```python
from build123d import *

# Parameters (mm, degrees)
BOSS_EXTRU_1_DEPTH      = 25
ESQUISSE6_W             = 10.8
ESQUISSE6_H             = 6
ENL_V_MAT_EXTRU_5_DEPTH = 16


with BuildPart() as part:
    # Esquisse1 → Boss.-Extru.1 (new body)
    with BuildSketch(Plane.XY):
        with BuildLine():
            Line((-2.515260994, 35.459016609), (-2.515260994, 31.759016609))
            ThreePointArc((-2.515260994, 31.759016609), (0.684739006, 30.959016609), (-2.515260994, 30.159016609))
            Line((-2.515260994, 30.159016609), (-2.515260994, -26.240983391))
            ThreePointArc((-2.515260994, -26.240983391), (0.684739006, -27.040983391), (-2.515260994, -27.840983391))
            Line((-2.515260994, -27.840983391), (-2.515260994, -40.420659447))
            ThreePointArc((-2.515260994, -40.420659447), (1.551219227, -35.231520618), (3, -28.8))
            Line((3, -28.8), (3, 32.7))
            ThreePointArc((3, 32.7), (1.706542051, 39.51560803), (-2.515260994, 45.020326491))
            Line((-2.515260994, 45.020326491), (-2.515260994, 35.459016609))
        make_face()
    extrude(amount=BOSS_EXTRU_1_DEPTH)

    # Esquisse6 → Enlèv. mat.-Extru.5 (cut)
    with BuildSketch(Plane(origin=(3, 0, 0), x_dir=(0, 0, -1), z_dir=(1, 0, 0))):
        with Locations((-12.5, 20.524263914)):
            Rectangle(ESQUISSE6_W, ESQUISSE6_H)
        with Locations((-12.5, -19.475736086)):
            Rectangle(ESQUISSE6_W, ESQUISSE6_H)
    extrude(amount=-ENL_V_MAT_EXTRU_5_DEPTH, mode=Mode.SUBTRACT)


solid = part.part
```
Input: part model. Units: mm. Frame: model coordinates. A direction names the side the tool comes from. Coordinates: 2 decimals unless noted, no trailing zeros. Order: outer loops, then holes, each group sorted by start corner. A loop starts at its lowest first (then second) coordinate and runs counter-clockwise, first axis right, second up. Notation, with made-up numbers: (75.25, -5.5) - (79.25, -5.5) arc R24 cw to (79.25, 11.5) - close; hole circle Ø3 at (70.25, -21.5). An arc over 180 degrees is marked (long way). Put each result on its own line as item: value.
1. Cut plane B-B on x = -1.8. Return the cut outline in (y, z).
Report:
outline: (-39.8, 0) - (-28.55, 0) - (-28.55, 25) - (-39.8, 25) - close; (-25.53, 0) - (29.45, 0) - (29.45, 25) - (-25.53, 25) - close; (32.47, 0) - (44.4, 0) - (44.4, 25) - (32.47, 25) - close; hole (-22.48, 7.1) - (-16.48, 7.1) - (-16.48, 17.9) - (-22.48, 17.9) - close; hole (17.52, 7.1) - (23.52, 7.1) - (23.52, 17.9) - (17.52, 17.9) - close
2. Line query: line 1 along Y through (x, z) = (1.7, 9); line 2 along Y through (x, z) = (-1.85, 5); line 3 along Y through (x, z) = (-1.8, 11.25). Output: solid intervals per line, ascending.
Report:
line 1: y = -34.91 to -22.48, -16.48 to 17.52, 23.52 to 39.53
line 2: y = -39.84 to -28.52, -25.56 to 29.48, 32.44 to 44.45
line 3: y = -39.8 to -28.55, -25.53 to -22.48, -16.48 to 17.52, 23.52 to 29.45, 32.47 to 44.4
3. Cut plane D-D on x = 1.9. Return the cut outline in (y, z), then the cut area to 3 significant figures.
Report:
outline: (-34.44, 0) - (39.06, 0) - (39.06, 25) - (-34.44, 25) - close; hole (-22.48, 7.1) - (-16.48, 7.1) - (-16.48, 17.9) - (-22.48, 17.9) - close; hole (17.52, 7.1) - (23.52, 7.1) - (23.52, 17.9) - (17.52, 17.9) - close
area: 1,710 mm2
4. Cut plane C-C on z = 19. Return the cut outline in (x, y), then the cut area to 3 significant figures.
Report:
outline: (-2.52, -40.42) arc R15 ccw to (3, -28.8) - (3, 32.7) arc R15 ccw to (-2.52, 45.02) - (-2.52, 31.76) arc R1.7 cw (long way) to (-2.52, 30.16) - (-2.52, -26.24) arc R1.7 cw (long way) to (-2.52, -27.84) - close
area: 415 mm2
5. Contact query for flat-ended pins moving along their axis: pin 1 Ø12.5 at (y, z) = (-10.5, 14.5) entering from +X; pin 2 Ø1.5 at (x, z) = (0.5, 18) entering from +Y; pin 3 Ø1.7 at (x, z) = (-0.5, 14) entering from +Y. Output: stop coordinate, or through.
Report:
pin 1: stops at x = 3
pin 2: stops at y = 42.73
pin 3: stops at y = 43.97
6. Reachability of faces 1 (the face through (0, -16.476, 13)), 2 (the face through (-2.515, 2, 12)) from +Z, -Z, +X, -X, +Y, -Y: full face, straight path, thin tool, end or side. Return the list, or none.
Report:
face 1: +X, -X
face 2: +Z, -Z, -X, +Y, -Y
7. Cut plane A-A on z = 9.75. Return the cut outline in (x, y), then the cut area to 3 significant figures.
Report:
outline: (-2.52, -40.42) arc R15 ccw to (3, -28.8) - (3, -22.48) - (-2.52, -22.48) - (-2.52, -26.24) arc R1.7 cw (long way) to (-2.52, -27.84) - close; (-2.52, -16.48) - (3, -16.48) - (3, 17.52) - (-2.52, 17.52) - close; (-2.52, 23.52) - (3, 23.52) - (3, 32.7) arc R15 ccw to (-2.52, 45.02) - (-2.52, 31.76) arc R1.7 cw (long way) to (-2.52, 30.16) - close
area: 348 mm2
8. Draft query along Y for faces 3 (the face through (1.51, -35.32, 12.32)), 4 (the face through (0, 17.524, 13)), 5 (the face through (0, 3, 25)). Return one class per face: pulls with the +Y half, pulls with the -Y half, needs draft (parallel to the pull), parting line crosses it, or undercut.
Report:
face 3: pulls with the -Y half
face 4: undercut
face 5: needs draft
